Input: part model. Units: mm. Frame: model coordinates. Face numbers are marked on the shaded views. A direction names the side the tool comes from. Give positions to 0.01 mm unless a question says otherwise; leave off trailing zeros. Loops run counter-clockwise (first coordinate to the right, second up) from the corner with the lowest first, then second, coordinate; pieces in that order, holes last. Notation, with made-up numbers: (32.5, -1.75) - (61.5, -1.75) arc R12 ccw to (61.5, 5.25) - close; hole circle Ø4 at (-32.75, 16). An arc over 180 degrees is marked (long way). One line per item, written item: value.
from build123d import *

# Parameters (mm, degrees)
SKETCH1_R           = 9
SKETCH1_R_2         = 3
BOSS_EXTRUDE1_DEPTH = 6
SKETCH2_R           = 7.25
SKETCH2_R_2         = 3
BOSS_EXTRUDE2_DEPTH = 11
SKETCH3_R           = 9
SKETCH3_R_2         = 3
BOSS_EXTRUDE3_DEPTH = 1
SKETCH4_R           = 1.5
CUT_EXTRUDE1_DEPTH  = 10


with BuildPart() as part:
    # Sketch1 → Boss-Extrude1 (new body)
    with BuildSketch(Plane.XY):
        Circle(SKETCH1_R)
        Circle(SKETCH1_R_2, mode=Mode.SUBTRACT)
    extrude(amount=BOSS_EXTRUDE1_DEPTH)

    # Sketch2 → Boss-Extrude2 (add)
    with BuildSketch(Plane.XY.offset(6)):
        Circle(SKETCH2_R)
        Circle(SKETCH2_R_2, mode=Mode.SUBTRACT)
    extrude(amount=BOSS_EXTRUDE2_DEPTH)

    # Sketch3 → Boss-Extrude3 (add)
    with BuildSketch(Plane.XY.offset(17)):
        Circle(SKETCH3_R)
        Circle(SKETCH3_R_2, mode=Mode.SUBTRACT)
    extrude(amount=BOSS_EXTRUDE3_DEPTH)

    # Sketch4 → Cut-Extrude1 (cut, through all)
    with BuildSketch(Plane(origin=(0, 0, 0), x_dir=(1, 0, 0), z_dir=(0, 1, 0))):
        with Locations((0, -4)):
            Circle(SKETCH4_R)
    extrude(amount=-CUT_EXTRUDE1_DEPTH, mode=Mode.SUBTRACT)


solid = part.part
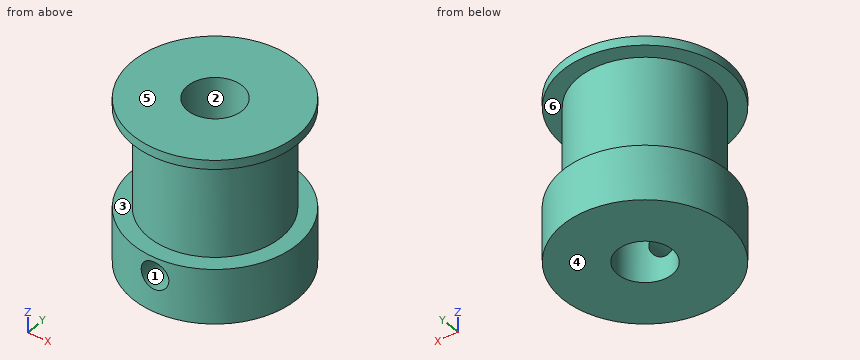
Item 1: Section B-B, the plane y = 0. Output: boundary loops of the cut face in (x, z).
Verdict:
outline: (-9, 0) - (-3, 0) - (-3, 18) - (-9, 18) - (-9, 17) - (-7.25, 17) - (-7.25, 6) - (-9, 6) - close; (3, 0) - (9, 0) - (9, 6) - (7.25, 6) - (7.25, 17) - (9, 17) - (9, 18) - (3, 18) - close
Item 2: Draft query along Z for the marked faces 4, 5 and 6. Return one class per face: pulls with the +Z half, pulls with the -Z half, needs draft (parallel to the pull), parting line crosses it, or undercut.
Verdict:
face 4: pulls with the -Z half
face 5: pulls with the +Z half
face 6: undercut
Item 3: Section C-C, the plane y = -3.5. Output: boundary loops of the cut face in (x, z).
Verdict:
outline: (-8.29, 0) - (8.29, 0) - (8.29, 6) - (6.35, 6) - (6.35, 17) - (8.29, 17) - (8.29, 18) - (-8.29, 18) - (-8.29, 17) - (-6.35, 17) - (-6.35, 6) - (-8.29, 6) - close; hole circle Ø3 at (0, 4)
Item 4: Access query for the marked faces 1, 2 and 3. Directions: +Z, -Z, +X, -X, +Y, -Y. A direction counts if a zero-diameter tool reaches every point of the face in a straight line with its end or side. Return the directions, or none.
Verdict:
face 1: -Y
face 2: +Z, -Z
face 3: none
Item 5: Material intervals for L1, parallel to Z at x = 8.25, y = 1.5; L2, parallel to Z at x = 0, y = -4.5; L3, parallel to X at y = -1.25, z = 15.75, sorted ascending.
Verdict:
L1: z = 0 to 6, 17 to 18
L2: z = 0 to 2.5, 5.5 to 18
L3: x = -7.14 to -2.73, 2.73 to 7.14
Item 6: Pin query (flat end, axial travel): P1, Ø6, axis at y = 3.5, z = 6, coming from the +X side; P2, Ø8, axis at x = -4, z = 6, coming from the +Y side; P3, Ø10, axis at y = -3, z = 11.5, coming from the -X side; P4, Ø3, axis at y = -1.5, z = 8, coming from the +X side. Return the tip coordinate at first contact, or that it passes through.
Verdict:
P1: stops at x = 8.99
P2: stops at y = 9
P3: stops at x = -7.25
P4: stops at x = 7.25
Item 7: Section A-A, the plane x = 0. Output: boundary loops of the cut face in (y, z), and give its area (4 significant figures).
Verdict:
outline: (-9, 0) - (-3, 0) - (-3, 2.5) - (-9, 2.5) - close; (-9, 5.5) - (-3, 5.5) - (-3, 18) - (-9, 18) - (-9, 17) - (-7.25, 17) - (-7.25, 6) - (-9, 6) - close; (3, 0) - (9, 0) - (9, 6) - (7.25, 6) - (7.25, 17) - (9, 17) - (9, 18) - (3, 18) - close
area: 159.5 mm^2
Item 8: Section D-D, the plane z = 13. Output: boundary loops of the cut face in (x, y).
Verdict:
outline: circle Ø14.5 at (0, 0); hole circle Ø6 at (0, 0)
